from build123d import *
from build123d.topology import SkipClean

# Parameters (mm, degrees)
SKETCH2_R           = 66.3
SKETCH2_R_2         = 62
BOSS_EXTRUDE1_DEPTH = 2
BOSS_EXTRUDE2_START = 6.5
BOSS_EXTRUDE2_DEPTH = 6.5


with BuildPart() as part:
    # Sketch2 → Boss-Extrude1 (new body)
    with BuildSketch(Plane(origin=(0, 0, 0), x_dir=(1, 0, 0), z_dir=(0, 1, 0))):
        with Locations(Location((0, 0, 0), (0, 0, 270))):
            Circle(SKETCH2_R)
        with Locations(Location((0, 0, 0), (0, 0, 270))):
            Circle(SKETCH2_R_2, mode=Mode.SUBTRACT)
    extrude(amount=BOSS_EXTRUDE1_DEPTH)

    # Sketch3 → Boss-Extrude2 (add)
    with SkipClean():  # the faces are left unmerged after this step: merging them gives an invalid solid
        with BuildSketch(Plane.XZ.offset(BOSS_EXTRUDE2_START)):
            with BuildLine():
                ThreePointArc((65.3, 0), (-46.174072811, -46.174072811), (0, 65.3))
                Line((0, 65.3), (0, 66.3))
                ThreePointArc((0, 66.3), (-46.881179593, -46.881179593), (66.3, 0))
                ThreePointArc((66.3, 0), (65.680309111, 9.043616265), (63.832820659, 17.918175317))
                Line((63.832820659, 17.918175317), (62.870033017, 17.647916262))
                ThreePointArc((62.870033017, 17.647916262), (64.689655881, 8.907211796), (65.3, 0))
            make_face()
        extrude(amount=-BOSS_EXTRUDE2_DEPTH)


solid = part.part
Source: CAD feature listing. Evaluate the final solid. Frame: model axes, mm. Round coordinates to 2 decimals unless told otherwise and drop trailing zeros. Loops run counter-clockwise (first coordinate to the right, second up) from the corner with the lowest first, then second, coordinate; pieces in that order, holes last. Notation, with made-up numbers: M -8,-20 L -3,-20 A21 ccw -3,-10 Z; hole C 19,69 d11. An arc over 180 degrees is marked long. Return JSON: item names as keys, results as strings. Group by question number.
1. Section query C-C on y = -4.5. Output: boundary loops of the cut face in (x, z).
2. Material intervals for line 1 along X through (y, z) = (0.9, 0); line 2 along Z through (x, y) = (-0.5, -1); line 3 along X through (y, z) = (-4, -18), sorted ascending. Write a range as from..to.
3. Mould query, pull axis Z, two halves, no side actions, for faces 1 (the face through (-44, 2, 44)), 2 (the face through (44, 0, 44)). Classes: released by +Z, released by -Z, zero draft, split by the parting line, or undercut.
4. Pin query (flat end, axial travel): pin 1 (5 mm diameter, centred on y = -0.5, z = 31.5, fed in from +X); pin 2 (4 mm diameter, centred on y = -0.5, z = 37, fed in from +X); pin 3 (3 mm diameter, centred on x = 41.5, y = 1, fed in from -Z). Return the tip coordinate at first contact, or that it passes through.
5. Section query D-D on z = 45. Output: boundary loops of the cut face in (x, y).
6. Section query A-A on z = -17.5. Output: boundary loops of the cut face in (x, y).
7. Section query B-B on x = -24. Output: boundary loops of the cut face in (y, z).
Checks:
{
 "1": {"outline": "M 0,65.3 L 0,66.3 A66.3 ccw long 63.83,17.92 L 62.87,17.65 A65.3 cw long Z"},
 "2": {"line 1": "x = -66.3..-62, 62..66.3", "line 2": "z = -66.3..-65.3, 65.3..66.3", "line 3": "x = -63.81..-62.77, 62.77..63.81"},
 "3": {"face 1": "zero draft", "face 2": "undercut"},
 "4": {"pin 1": "stops at x = 59.6", "pin 2": "stops at x = 56.27", "pin 3": "stops at z = -52.87"},
 "5": {"outline": "M -48.69,-6.5 L -47.32,-6.5 L -47.32,0 L -42.65,0 L -42.65,2 L -48.69,2 Z; M 42.65,0 L 48.69,0 L 48.69,2 L 42.65,2 Z"},
 "6": {"outline": "M -63.95,-6.5 L -62.91,-6.5 L -62.91,0 L -59.48,0 L -59.48,2 L -63.95,2 Z; M 59.48,0 L 62.91,0 L 62.91,-6.5 L 63.95,-6.5 L 63.95,2 L 59.48,2 Z"},
 "7": {"outline": "M -6.5,-61.8 L 2,-61.8 L 2,-57.17 L 0,-57.17 L 0,-60.73 L -6.5,-60.73 Z; M -6.5,60.73 L 0,60.73 L 0,57.17 L 2,57.17 L 2,61.8 L -6.5,61.8 Z"}
}
